Build history of the part. All positions in model axes, mm. Face numbers are marked on the shaded views. A direction names the side the tool comes from. Round coordinates to 2 decimals unless told otherwise and drop trailing zeros. Write each loop counter-clockwise with the first axis right and the second up, starting at its lowest first coordinate (ties: lowest second). Pieces come first, ordered by that corner, then holes. Notation, with made-up numbers: (-24.75, -25) - (0.25, -25) arc R37 cw to (0.25, 12) - close; hole circle Ø3 at (67.5, 30.25). An arc over 180 degrees is marked (long way). Answer as a JSON object with one key per item and string values. Group by question number.
Item 1: Slice it at C-C, the plane x = 2.25. List the corners of the cut face in (y, z), then the cut area to 3 significant figures.
Item 2: Slice it at D-D, the plane y = -16. List the corners of the cut face in (x, z), then the cut area to 3 significant figures.
Item 3: Probe line 1 (Y direction, x = 8, z = 5.05); line 2 (X direction, y = 4.5, z = 5.3); line 3 (X direction, y = 4.5, z = 5.65). List the from-to ranges inside material, lowest first. Write a range as from..to.
Item 4: Slice it at B-B, the plane y = 16. List the corners of the cut face in (x, z), then the cut area to 3 significant figures.
Item 5: Flat gauge pins, fed straight in: pin 1 (2 mm diameter, centred on x = 1.5, y = 14, fed in from +Z); pin 2 (4.5 mm diameter, centred on x = -9, y = 5, fed in from +Z); pin 3 (3 mm diameter, centred on x = -8, y = 4.5, fed in from -Z). Where does each tip first touch, or does it go through?
Item 6: Which spindle directions (+Z, -Z, +X, -X, +Y, -Y) get a long thin tool onto all of the face, cutting with end or side? Do the marked faces 1, 2, 3, 4 and 5. Say none if no direction does.
Item 7: Slice it at A-A, the plane z = 0. List the corners of the cut face in (x, y), then the cut area to 3 significant figures.
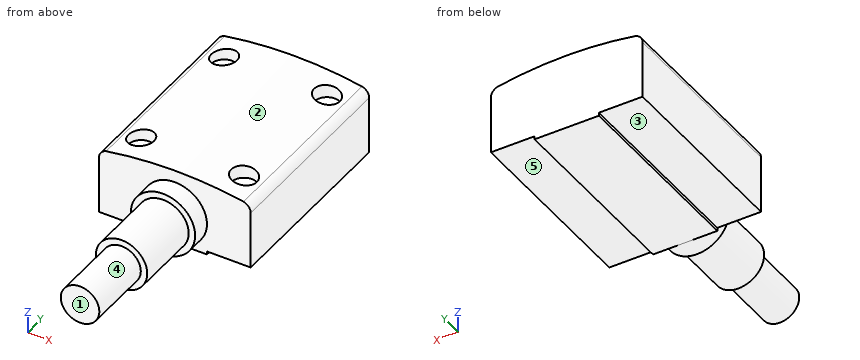
from build123d import *

# Parameters (mm, degrees)
SKETCH_1_W          = 10
SKETCH_1_H          = 0.5
EXTRUDE_3_DEPTH     = 30
SKETCH_4_R          = 5
EXTRUDE_4_DEPTH     = 3
SKETCH_5_R          = 4
EXTRUDE_5_DEPTH     = 10.5
SKETCH_6_R          = 3
EXTRUDE_6_DEPTH     = 10.5
CUT_EXTRUDE_2_REACH = 4.408
SKETCH_9_R          = 2


with BuildPart() as part:
    # ｽｹｯﾁ1 → ﾎﾞｽ - 押し出し3 (new body)
    with BuildSketch(Plane(origin=(0, 0, 0), x_dir=(1, 0, 0), z_dir=(0, 1, 0))):
        with BuildLine():
            Line((-5, 4.5), (-11.8, 4.5))
            Line((-11.8, 4.5), (-11.8, -4.5))
            Line((-11.8, -4.5), (0, -4.5))
            ThreePointArc((0, -4.5), (-3.535533906, -3.035533906), (-5, 0.5))
            Line((-5, 0.5), (-5, 4.5))
        make_face()
        with BuildLine():
            Line((5, 4.5), (-5, 4.5))
            Line((-5, 4.5), (-5, 0.5))
            ThreePointArc((-5, 0.5), (-3.535533906, -3.035533906), (0, -4.5))
            ThreePointArc((0, -4.5), (3.535533906, -3.035533906), (5, 0.5))
            Line((5, 0.5), (5, 4.5))
        make_face()
        with BuildLine():
            Line((11.8, 4.5), (5, 4.5))
            Line((5, 4.5), (5, 0.5))
            ThreePointArc((5, 0.5), (3.535533906, -3.035533906), (0, -4.5))
            Line((0, -4.5), (11.8, -4.5))
            Line((11.8, -4.5), (11.8, 4.5))
        make_face()
        with BuildLine():
            ThreePointArc((-11.8, -4.5), (-11.49003001, -5.413142144), (-10.688228568, -5.948888739))
            ThreePointArc((-10.688228568, -5.948888739), (0, -6.908263067), (10.688228568, -5.948888739))
            ThreePointArc((10.688228568, -5.948888739), (11.49003001, -5.413142144), (11.8, -4.5))
            Line((11.8, -4.5), (-11.8, -4.5))
        make_face()
        with Locations((0, 4.75)):
            Rectangle(SKETCH_1_W, SKETCH_1_H)
    extrude(amount=EXTRUDE_3_DEPTH)

    # ｽｹｯﾁ4 → ﾎﾞｽ - 押し出し4 (add)
    with BuildSketch(Plane.XZ):
        Circle(SKETCH_4_R)
    extrude(amount=EXTRUDE_4_DEPTH)

    # ｽｹｯﾁ5 → ﾎﾞｽ - 押し出し5 (add)
    with BuildSketch(Plane.XZ.offset(3)):
        Circle(SKETCH_5_R)
    extrude(amount=EXTRUDE_5_DEPTH)

    # ｽｹｯﾁ6 → ﾎﾞｽ - 押し出し6 (add)
    with BuildSketch(Plane.XZ.offset(13.5)):
        Circle(SKETCH_6_R)
    extrude(amount=EXTRUDE_6_DEPTH)

    # ｽｹｯﾁ9 → ｶｯﾄ - 押し出し2 (cut, up to next)
    with BuildSketch(Plane(origin=(0, 0, 4.5), x_dir=(-1, 0, 0), z_dir=(0, 0, -1)), mode=Mode.PRIVATE) as cut_extrude_2_sk1:
        with Locations((-8, 4.5)):
            Circle(SKETCH_9_R)
    cut_extrude_2_tool1 = extrude(cut_extrude_2_sk1.sketch, amount=-CUT_EXTRUDE_2_REACH, mode=Mode.PRIVATE) & part.part
    add(cut_extrude_2_tool1.solids().sort_by_distance((8, 4.5, 4.5))[0], mode=Mode.SUBTRACT)
    # ｽｹｯﾁ9 → ｶｯﾄ - 押し出し2 (cut, up to next)
    with BuildSketch(Plane(origin=(0, 0, 4.5), x_dir=(-1, 0, 0), z_dir=(0, 0, -1)), mode=Mode.PRIVATE) as cut_extrude_2_sk2:
        with Locations((8, 4.5)):
            Circle(SKETCH_9_R)
    cut_extrude_2_tool2 = extrude(cut_extrude_2_sk2.sketch, amount=-CUT_EXTRUDE_2_REACH, mode=Mode.PRIVATE) & part.part
    add(cut_extrude_2_tool2.solids().sort_by_distance((-8, 4.5, 4.5))[0], mode=Mode.SUBTRACT)
    # ｽｹｯﾁ9 → ｶｯﾄ - 押し出し2 (cut, up to next)
    with BuildSketch(Plane(origin=(0, 0, 4.5), x_dir=(-1, 0, 0), z_dir=(0, 0, -1)), mode=Mode.PRIVATE) as cut_extrude_2_sk3:
        with Locations((8, 25.5)):
            Circle(SKETCH_9_R)
    cut_extrude_2_tool3 = extrude(cut_extrude_2_sk3.sketch, amount=-CUT_EXTRUDE_2_REACH, mode=Mode.PRIVATE) & part.part
    add(cut_extrude_2_tool3.solids().sort_by_distance((-8, 25.5, 4.5))[0], mode=Mode.SUBTRACT)
    # ｽｹｯﾁ9 → ｶｯﾄ - 押し出し2 (cut, up to next)
    with BuildSketch(Plane(origin=(0, 0, 4.5), x_dir=(-1, 0, 0), z_dir=(0, 0, -1)), mode=Mode.PRIVATE) as cut_extrude_2_sk4:
        with Locations((-8, 25.5)):
            Circle(SKETCH_9_R)
    cut_extrude_2_tool4 = extrude(cut_extrude_2_sk4.sketch, amount=-CUT_EXTRUDE_2_REACH, mode=Mode.PRIVATE) & part.part
    add(cut_extrude_2_tool4.solids().sort_by_distance((8, 25.5, 4.5))[0], mode=Mode.SUBTRACT)


solid = part.part
Geometry says:
{
 "1": {"outline": "(-24, -1.98) - (-13.5, -1.98) - (-13.5, -3.31) - (-3, -3.31) - (-3, -4.47) - (0, -4.47) - (0, -5) - (30, -5) - (30, 6.87) - (0, 6.87) - (0, 4.47) - (-3, 4.47) - (-3, 3.31) - (-13.5, 3.31) - (-13.5, 1.98) - (-24, 1.98) - close", "area": "494 mm^2"},
 "2": {"outline": "circle Ø6 at (0, 0)", "area": "28.3 mm^2"},
 "3": {"line 1": "y = 0..2.5, 6.5..23.5, 27.5..30", "line 2": "x = -11.57..-10, -6..6, 10..11.57", "line 3": "x = -11.26..-10, -6..6, 10..11.26"},
 "4": {"outline": "(-11.8, -4.5) - (-5, -4.5) - (-5, -5) - (5, -5) - (5, -4.5) - (11.8, -4.5) - (11.8, 4.5) arc R1.5 ccw to (10.69, 5.95) arc R60.02 ccw to (-10.69, 5.95) arc R1.5 ccw to (-11.8, 4.5) - close", "area": "264 mm^2"},
 "5": {"pin 1": "stops at z = 6.91", "pin 2": "stops at z = 6.48", "pin 3": "stops at z = -4.5"},
 "6": {"face 1": "+Z, -Z, +X, -X, -Y", "face 2": "+Z, +Y, -Y", "face 3": "-Z, -X, +Y, -Y", "face 4": "-Y", "face 5": "-Z, +X, +Y, -Y"},
 "7": {"outline": "(-11.8, 0) - (-5, 0) - (-5, -3) - (-4, -3) - (-4, -13.5) - (-3, -13.5) - (-3, -24) - (3, -24) - (3, -13.5) - (4, -13.5) - (4, -3) - (5, -3) - (5, 0) - (11.8, 0) - (11.8, 30) - (-11.8, 30) - close", "area": "885 mm^2"}
}
